For this review, use the dimensioned drawing (mm, ordinates from the lowest corner) and the shaded views. A direction names the side the tool comes from. Give positions to 0.01 mm unless a question says otherwise; leave off trailing zeros. Loops run counter-clockwise (first coordinate to the right, second up) from the corner with the lowest first, then second, coordinate; pieces in that order, holes last. Notation, with made-up numbers: (-23, -38) -> (-3, -38) arc R21 ccw to (-3, -29) -> close; hole circle Ø1 at (77.5, 33.5). An arc over 180 degrees is marked (long way). Write each question's results on one line, items separated by ' | '. Start each with the question number.
Q1. Machinability: for the marked faces 5, 6, 7, 8 and 9, which of the approach directions +Z, -Z, +X, -X, +Y, -Y give a long, thin tool a straight path to every point of the face, cutting with its end or side? Answer none if there is none.
Q2. We need section D-D (x = 10). Write out the cut boundary in (y, z), plus the area to 3 significant figures.
Q3. We need section C-C (z = 10.25). Write out the cut boundary in (x, y), plus the area to 3 significant figures.
Q4. Insertion check: pin 1 Ø3 at (x, z) = (11.5, 2) entering from -Y; pin 2 Ø6 at (x, z) = (13.5, 3.5) entering from +Y; pin 3 Ø10 at (y, z) = (65, 20.5) entering from -X. Each pin has a flat end and moves straight along its axis. Give the tip position at first contact, or say it passes through.
Q5. Mouldability with a two-part tool opening along X and no side actions: class the marked faces 1, 2, 3 and 4 as released by +X, released by -X, zero draft, split by the parting line, or undercut.
Q6. We need section A-A (z = 1.5). Write out the cut boundary in (x, y) (3 decimals), plus the area to 3 significant figures.
Q7. Wall thickness on L1, parallel to X at y = 67.5, z = 3.75; L2, parallel to Z at x = 32, y = 12; L3, parallel to Y at x = 63, z = 3: over which ranges is each line inside the solid? List them lowest first. Write a range as [from, to].
Q8. We need section B-B (y = 38.1). Write out the cut boundary in (x, z).
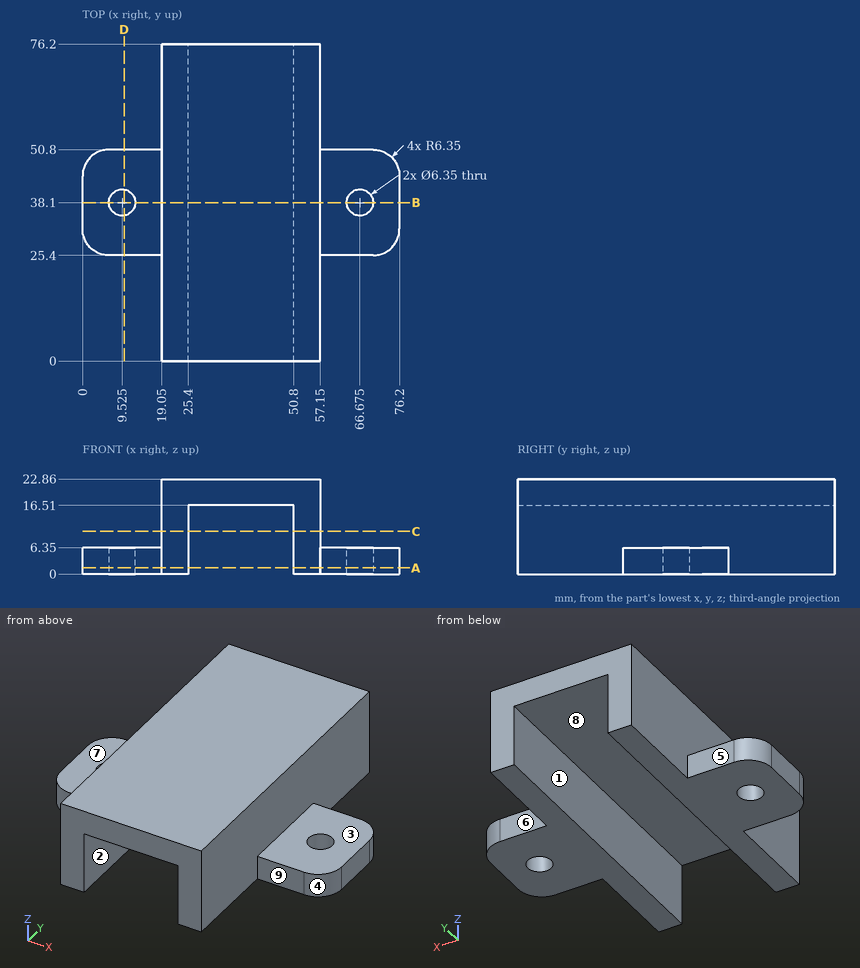
Output:
1) face 5: +Z, -Z, -X, +Y | face 6: +Z, -Z, +X, +Y | face 7: +Z, -X, +Y, -Y | face 8: -Z, +Y, -Y | face 9: +Z, -Z, +X, -Y
2) outline: (25.4, 0) -> (34.96, 0) -> (34.96, 6.35) -> (25.4, 6.35) -> close; (41.24, 0) -> (50.8, 0) -> (50.8, 6.35) -> (41.24, 6.35) -> close | area: 121 mm2
3) outline: (19.05, 0) -> (25.4, 0) -> (25.4, 76.2) -> (19.05, 76.2) -> close; (50.8, 0) -> (57.15, 0) -> (57.15, 76.2) -> (50.8, 76.2) -> close | area: 968 mm2
4) pin 1: y = 25.4 | pin 2: y = 50.8 | pin 3: x = 19.05
5) face 1: undercut | face 2: undercut | face 3: zero draft | face 4: released by +X
6) outline: (0, 31.75) arc R6.35 ccw to (6.35, 25.4) -> (19.05, 25.4) -> (19.05, 0) -> (25.4, 0) -> (25.4, 76.2) -> (19.05, 76.2) -> (19.05, 50.8) -> (6.35, 50.8) arc R6.35 ccw to (0, 44.45) -> close; (50.8, 0) -> (57.15, 0) -> (57.15, 25.4) -> (69.85, 25.4) arc R6.35 ccw to (76.2, 31.75) -> (76.2, 44.45) arc R6.35 ccw to (69.85, 50.8) -> (57.15, 50.8) -> (57.15, 76.2) -> (50.8, 76.2) -> close; hole circle Ø6.35 at (9.525, 38.1); hole circle Ø6.35 at (66.675, 38.1) | area: 1,840 mm2
7) L1: [19.05, 25.4], [50.8, 57.15] | L2: [16.51, 22.86] | L3: [25.4, 50.8]
8) outline: (0, 0) -> (6.35, 0) -> (6.35, 6.35) -> (0, 6.35) -> close; (12.7, 0) -> (25.4, 0) -> (25.4, 16.51) -> (50.8, 16.51) -> (50.8, 0) -> (63.5, 0) -> (63.5, 6.35) -> (57.15, 6.35) -> (57.15, 22.86) -> (19.05, 22.86) -> (19.05, 6.35) -> (12.7, 6.35) -> close; (69.85, 0) -> (76.2, 0) -> (76.2, 6.35) -> (69.85, 6.35) -> close
